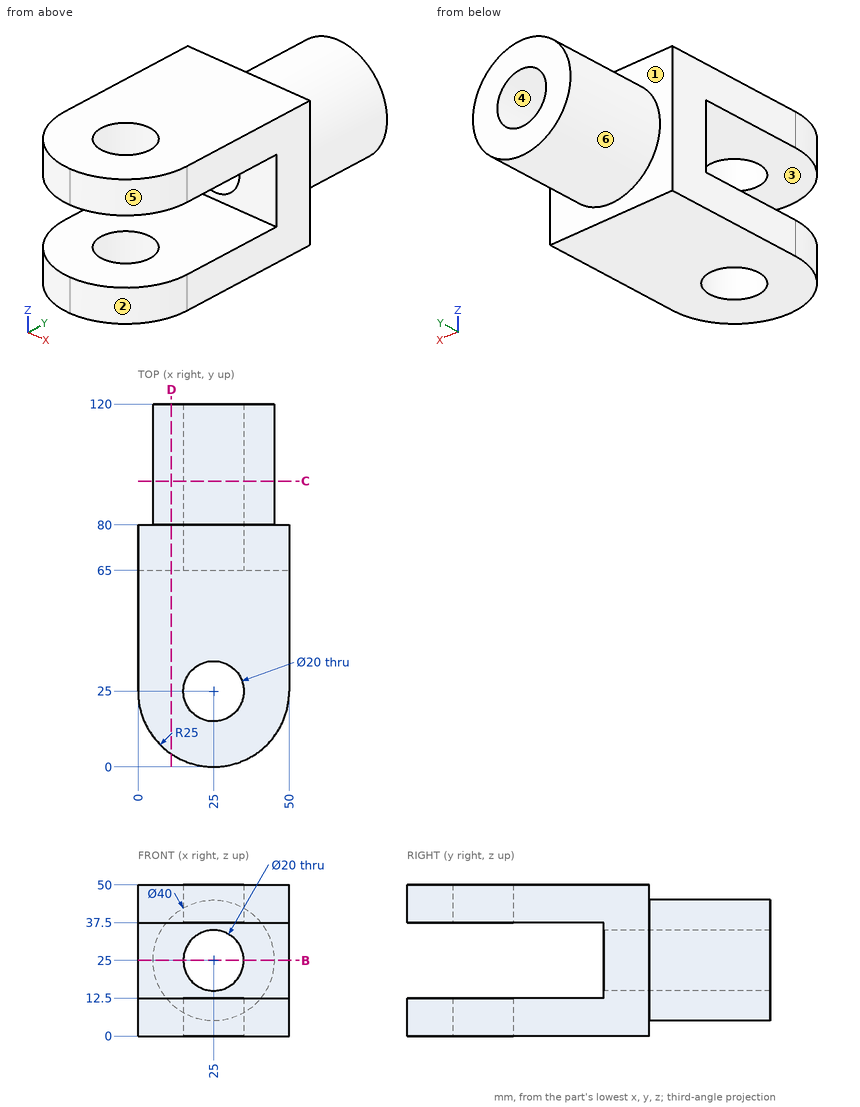
For this review, use the dimensioned drawing (mm, ordinates from the lowest corner) and the shaded views. A direction names the side the tool comes from. Give positions to 0.01 mm unless a question says otherwise; leave off trailing zeros. Loops run counter-clockwise (first coordinate to the right, second up) from the corner with the lowest first, then second, coordinate; pieces in that order, holes last. Notation, with made-up numbers: (81.25, 63) -> (110.25, 63) arc R21 ccw to (110.25, 96) -> close; hole circle Ø3 at (-32, 82.5). An arc over 180 degrees is marked (long way). One line per question, with ' | ' between items. Start each with the question number.
(1) For the marked faces 1, 2 and 3, list the 3-axis set-ups (+Z, -Z, +X, -X, +Y, -Y) from which the entire face can be reached by the end or side of a thin tool; tool diameter is ignored.
(2) Draft analysis for pull direction Z (two halves, no side actions). For the marked faces 4, 5 and 6, state which applies: +Z half, -Z half, draft (parallel to the pull), parting line (faces both ways), or undercut.
(3) We need section D-D (x = 11). State the section outline as (y, z) points.
(4) We need section C-C (y = 94.5). State the section outline as (x, z) points.
(5) Insertion check: P1, Ø12, axis at x = 25, y = 25, coming from the +Z side; P2, Ø10, axis at x = 15.5, z = 18, coming from the -Y side; P3, Ø1.5, axis at x = 17, z = 12, coming from the -Y side. Each pin has a flat end and moves straight along its axis. Give the tip position at first contact, or say it passes through.
(6) For line 1 (Z direction, x = 12, y = 14.5); line 2 (Z direction, x = 25, y = 93); line 3 (Y direction, x = 37.5, z = 21.5), list the stretches that pass through material, from the lowest coordinate up.
(7) We need section B-B (z = 25). State the section outline as (x, y) points.
The answers:
1) face 1: +Y | face 2: +Z, -Z, +X, -Y | face 3: +X, -X, -Y
2) face 4: undercut | face 5: draft | face 6: parting line
3) outline: (4.29, 0) -> (80, 0) -> (80, 10.72) -> (120, 10.72) -> (120, 39.28) -> (80, 39.28) -> (80, 50) -> (4.29, 50) -> (4.29, 37.5) -> (65, 37.5) -> (65, 12.5) -> (4.29, 12.5) -> close
4) outline: circle Ø40 at (25, 25); hole circle Ø20 at (25, 25)
5) P1: passes through | P2: stops at y = 65 | P3: stops at y = 1.07
6) line 1: z = 0 to 12.5, 37.5 to 50 | line 2: z = 5 to 15, 35 to 45 | line 3: y = 65 to 120
7) outline: (0, 65) -> (15, 65) -> (15, 120) -> (5, 120) -> (5, 80) -> (0, 80) -> close; (35, 65) -> (50, 65) -> (50, 80) -> (45, 80) -> (45, 120) -> (35, 120) -> close
